Source: CAD feature listing. Evaluate the final solid. Frame: model axes, mm. Give positions to 0.01 mm unless a question says otherwise; leave off trailing zeros. Order: outer loops, then holes, each group sorted by start corner. A loop starts at its lowest first (then second) coordinate and runs counter-clockwise, first axis right, second up.
Autodesk Inventor part; units mm, degrees
ref_plane "Work Plane1" through (6.4265, 6.5449, 0) normal (1, 0, 0) x (0, 1, 0)
ref_plane "XZ Plane" through (0, 0, 0) normal (0, 1, 0) x (-1, 0, 0)
ref_plane "XY Plane" through (0, 0, 0) normal (0, 0, 1) x (1, 0, 0)
sketch "Sketch1" plane through (0, 0, 0) normal (0, 0, 1) x (1, 0, 0)
  circle A0 centre (-10.274, 6.5449) radius 16.7005
  dimension "d0" = 33.401
extrude "Extrusion1" add sketch "Sketch1" along normal blind 520.7
shell "Shell1" thickness 3.3782 removed faces 2 at (-15.0414, 5.2901, 0) at (-15.0414, 5.2901, 520.7)
ref_plane "Work Plane1" through (6.4265, 6.5449, 0) normal (1, 0, 0) x (0, 1, 0)
sketch "Sketch3" plane through (6.4265, 6.5449, 0) normal (1, 0, 0) x (0, 1, 0)
  line L0 (13.3223, 0) -> (-13.3223, 0)
  circle A0 centre (0, 9.525) radius 6.35
  dimension "d4" = 12.7
  dimension "d5" = 9.525
extrude "Extrusion2" cut sketch "Sketch3" against normal through all
properties part number "FE-00003-01"
1) Ray query, L1, parallel to X at y = 5.5, z = 418.5; L2, parallel to Y at x = -10.5, z = 173; L3, parallel to X at y = 18, z = 248. Return the intervals inside material, ascending.
Checks:
L1: x = -26.94 to -23.56, 3.01 to 6.39
L2: y = -10.15 to -6.78, 19.87 to 23.24
L3: x = -22.43 to -17.08, -3.47 to 1.88
2) Section query B-B on z = 100. Output: boundary loops of the cut face in (x, y), and give its area (3 significant figures).
Checks:
outline: circle Ø33.4 at (-10.27, 6.54); hole circle Ø26.64 at (-10.27, 6.54)
area: 319 mm2
3) Pull-direction query (Y, two-part tool) for faces 1 (the face through (-23, 2, 520.7)), 2 (the face through (-24.445, 1.506, 5.661)), 3 (the face through (5.655, 1.529, 256.705)); classes: +Y half, -Y half, draft (parallel to the pull), parting line (faces both ways), or undercut.
Checks:
face 1: draft
face 2: undercut
face 3: parting line
4) First-contact query: pin 1 Ø1.5 at (y, z) = (11.5, 292) entering from -X; pin 2 Ø3 at (x, z) = (-16, 162.5) entering from -Y; pin 3 Ø1.5 at (x, z) = (-12, 162) entering from -Y; pin 4 Ø3 at (x, y) = (-5.5, -3.5) entering from -Z. Flat tips, straight axial feed; report the tip coordinate or a pass-through.
Checks:
pin 1: stops at x = -26.44
pin 2: stops at y = -9.61
pin 3: stops at y = -10.13
pin 4: passes through
5) Section query A-A on x = -3.5. Output: boundary loops of the cut face in (y, z), and give its area (3 significant figures).
Checks:
outline: (-8.72, 0) - (-4.93, 0) - (-4.93, 520.7) - (-8.72, 520.7) - close; (18.02, 0) - (21.81, 0) - (21.81, 520.7) - (18.02, 520.7) - close
area: 3,950 mm2
